The model under review builds one solid part; all positions refer to its coordinate system, in mm. A direction names the side the tool comes from. Round coordinates to 2 decimals unless told otherwise and drop trailing zeros. Order: outer loops, then holes, each group sorted by start corner. A loop starts at its lowest first (then second) coordinate and runs counter-clockwise, first axis right, second up. Notation, with made-up numbers: (87.5, -33.5) - (115.5, -33.5) arc R28 cw to (115.5, -10.5) - close; hole circle Ø2 at (74, 19.25). An arc over 180 degrees is marked (long way). One line per question, with ' | ' between items. Start each with the question number.
Item 1: Tool access review of faces 4 (the face through (9.54, -3, 12.85)), 5 (the face through (-0.521, 19.437, 13.966)), 6 (the face through (-19.437, -0.521, 13.966)): name each direction out of +Z, -Z, +X, -X, +Y, -Y from which nothing blocks a thin tool from reaching the whole face with its end or side.
Item 2: Add section B-B on y = 0. State the section outline as (x, z) points, and give its area (3 significant figures).
Item 3: Add section A-A on x = 0. State the section outline as (y, z) points, and give its area (3 significant figures).
Item 4: Add section D-D on z = 63. State the section outline as (x, y) points.
Item 5: Insertion check: pin 1 Ø10 at (x, z) = (-8, 21) entering from +Y; pin 2 Ø10 at (y, z) = (-21, 33) entering from +X; pin 3 Ø2 at (x, z) = (-22, 81) entering from -Y; pin 4 Ø13 at (x, z) = (0, 10) entering from +Y. Each pin has a flat end and moves straight along its axis. Give the tip position at first contact, or say it passes through.
Item 6: For L1, parallel to Y at x = 0, z = 19; L2, parallel to Z at x = 0, y = 14.5; L3, parallel to X at y = 0, z = 11, list the stretches that pass through material, from the lowest coordinate up. Write a range as [from, to].
Item 7: Add section C-C on z = 10. State the section outline as (x, y) points, and give its area (3 significant figures).
Item 8: Draft analysis for pull direction X (two halves, no side actions). For faces 1 (the face through (27.712, -11.49, 50.314)), 2 (the face through (0, 0, 100)), 3 (the face through (0, 0, 24)), state which applies: +X half, -X half, draft (parallel to the pull), parting line (faces both ways), or undercut.
from build123d import *

# Parameters (mm, degrees)
F0_R     = 30
F1_DEPTH = 100
F2_R     = 10
F3_DEPTH = 24
F4_R     = 2
F5_R     = 4
F6_DEPTH = 30
F7_R     = 4
F8_DEPTH = 30


with BuildPart() as f1:
    # F0 (on Top) → F1 (new body)
    with BuildSketch(Plane.XY):
        Circle(F0_R)
    extrude(amount=F1_DEPTH)

    # F2 (on face) → F3 (cut)
    with BuildSketch(Plane(origin=(0, 0, 0), x_dir=(1, 0, 0), z_dir=(0, 0, -1))):
        Circle(F2_R)
    extrude(amount=-F3_DEPTH, mode=Mode.SUBTRACT)

    # F4
    f4_edges = [f1.edges().sort_by_distance(p)[0] for p in [
        (-10, 0, 0),
        (-30, 0, 0),
    ]]
    fillet(f4_edges, radius=F4_R)

    # F5 (on Right) → F6 (cut)
    with BuildSketch(Plane.YZ):
        with Locations((0, 10)):
            Circle(F5_R)
    extrude(amount=-F6_DEPTH, mode=Mode.SUBTRACT)

    # F7 (on Front) → F8 (cut)
    with BuildSketch(Plane.XZ):
        with Locations((0, 10)):
            Circle(F7_R)
    extrude(amount=-F8_DEPTH, mode=Mode.SUBTRACT)


solid = f1.part
Determined:
1) face 4: -Z | face 5: +Y | face 6: -X
2) outline: (-30, 2) arc R2 ccw to (-28, 0) - (-12, 0) arc R2 ccw to (-10, 2) - (-10, 6) - (-30, 6) - close; (-30, 14) - (-10, 14) - (-10, 24) - (10, 24) - (10, 2) arc R2 ccw to (12, 0) - (28, 0) arc R2 ccw to (30, 2) - (30, 100) - (-30, 100) - close | area: 5,360 mm2
3) outline: (-30, 2) arc R2 ccw to (-28, 0) - (-12, 0) arc R2 ccw to (-10, 2) - (-10, 24) - (10, 24) - (10, 14) - (30, 14) - (30, 100) - (-30, 100) - close; (10, 2) arc R2 ccw to (12, 0) - (28, 0) arc R2 ccw to (30, 2) - (30, 6) - (10, 6) - close | area: 5,360 mm2
4) outline: circle Ø60 at (0, 0)
5) pin 1: y = 29.85 | pin 2: x = 25.38 | pin 3: y = -21.42 | pin 4: y = 30
6) L1: [-30, -10], [10, 30] | L2: [0, 6], [14, 100] | L3: [10, 30]
7) outline: (-29.73, -4) arc R30 ccw (long way) to (4, 29.73) - (4, 9.17) arc R10 cw (long way) to (-9.17, -4) - close; (-29.73, 4) - (-9.17, 4) arc R10 cw to (-4, 9.17) - (-4, 29.73) arc R30 ccw to start | area: 2,190 mm2
8) face 1: parting line | face 2: draft | face 3: undercut
